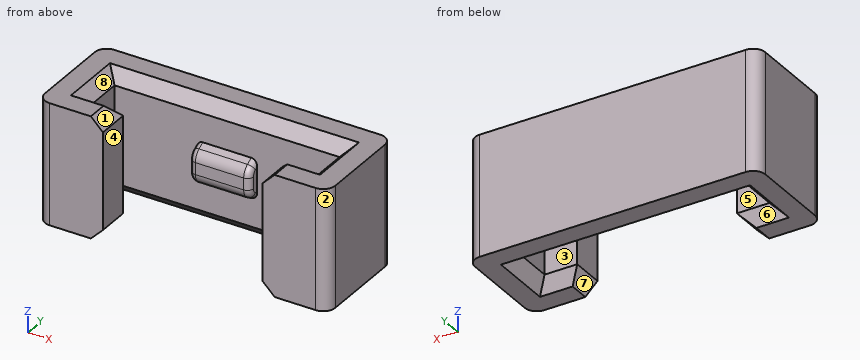
from build123d import *

# Parameters (mm, degrees)
F1_DEPTH    = 10
F2_W        = 5
F2_H        = 3.4
F3_DEPTH    = 1
F4_T4_DEPTH = 10.6915886602
F4_T9_DEPTH = 10.6915886602
F5_R        = 1
F6_R        = 0.5
F7_SIZE     = 1
F8_R        = 1


# Not quite as in the source:
# - a fillet or chamfer that OpenCascade refuses, or shapes differently, is made with other operations: its cross-section is extruded or revolved along the edge and cut away or added


with BuildPart() as f1:
    # F0 (on Top) → F1 (new body)
    with BuildSketch(Plane.XY):
        Polygon((-6.6, -5.9), (-9.3, -5.9), (-9.3, -2.7), (0, -2.7), (9.3, -2.7), (9.3, -5.9), (6.6, -5.9), (6.6, -8.6), (12, -8.6), (12, 0), (0, 0), (-12, 0), (-12, -8.6), (-6.6, -8.6), align=None)
    extrude(amount=F1_DEPTH)

    # F2 (on face) → F3 (join)
    with BuildSketch(Plane.XZ.offset(2.7)):
        with Locations((0, 5)):
            Rectangle(F2_W, F2_H)
    extrude(amount=F3_DEPTH)

    # F4: chamfer of 1.1 x 0.6350852961 on 2 edges, made by hand


with BuildPart() as f4_tool2:
    # F4_s3 → F4_t4 (new body)
    with BuildSketch(Plane.YZ.offset(5.3457943301)):
        Polygon((-2.6, 6.7), (-3.7, 6.0649147039), (-3.7, 6.7), align=None)
    extrude(amount=-F4_T4_DEPTH)

    split(bisect_by=Plane.XZ.offset(2.7), keep=Keep.TOP)


with BuildPart() as f1_1:
    add(f1.part)

    # F4_t1: cut F4_tool2
    add(f4_tool2.part, mode=Mode.SUBTRACT)


with BuildPart() as f4_tool7:
    # F4_s8 → F4_t9 (new body)
    with BuildSketch(Plane.YZ.offset(-5.3457943301)):
        Polygon((-2.6, 3.3), (-3.7, 3.9350852961), (-3.7, 3.3), align=None)
    extrude(amount=F4_T9_DEPTH)

    split(bisect_by=Plane.XZ.offset(2.7), keep=Keep.TOP)


with BuildPart() as f1_2:
    add(f1_1.part)

    # F4_t6: cut F4_tool7
    add(f4_tool7.part, mode=Mode.SUBTRACT)

    # F5
    f5_edges = [f1_2.edges().sort_by_distance(p)[0] for p in [
        (0, -3.7, 3.935085),
        (0, -3.7, 6.064915),
    ]]
    fillet(f5_edges, radius=F5_R)

    # F6
    f6_edges = [f1_2.edges().sort_by_distance(p)[0] for p in [
        (2.5, -3.566025, 4.012436),
        (2.5, -3.566025, 5.987564),
        (-2.5, -3.566025, 4.012436),
        (-2.5, -3.566025, 5.987564),
        (2.5, -2.95, 6.497927),
        (-2.5, -2.95, 6.497927),
        (2.5, -3.7, 5),
        (2.5, -2.95, 3.502073),
        (-2.5, -2.95, 3.502073),
        (-2.5, -3.7, 5),
    ]]
    fillet(f6_edges, radius=F6_R)

    # F7
    f7_edges = [f1_2.edges().sort_by_distance(p)[0] for p in [
        (-9.3, -4.3, 0),
        (0, -2.7, 0),
        (-7.95, -5.9, 0),
        (-6.6, -7.25, 0),
        (9.3, -4.3, 0),
        (7.95, -5.9, 0),
        (6.6, -7.25, 0),
        (-9.3, -4.3, 10),
        (-7.95, -5.9, 10),
        (-6.6, -7.25, 10),
        (0, -2.7, 10),
        (9.3, -4.3, 10),
        (7.95, -5.9, 10),
        (6.6, -7.25, 10),
    ]]
    chamfer(f7_edges, length=F7_SIZE)

    # F8
    f8_edges = [f1_2.edges().sort_by_distance(p)[0] for p in [
        (-12, -8.6, 5),
        (12, -8.6, 5),
        (-12, 0, 5),
        (12, 0, 5),
    ]]
    fillet(f8_edges, radius=F8_R)


solid = f1_2.part
Source: CAD feature listing. Evaluate the final solid. Frame: model axes, mm. Face numbers are marked on the shaded views. A direction names the side the tool comes from. Round coordinates to 2 decimals unless told otherwise and drop trailing zeros. Loops run counter-clockwise (first coordinate to the right, second up) from the corner with the lowest first, then second, coordinate; pieces in that order, holes last. Notation, with made-up numbers: (6.25, 75.5) -> (44.25, 75.5) arc R10 cw to (44.25, 93.5) -> close; hole circle Ø3 at (17.25, 71). An arc over 180 degrees is marked (long way). Answer as a JSON object with one key per item and string values. Group by question number.
Q1. Section query B-B (y = -4.75). Output: boundary loops of the cut face in (x, z), plus the area to 3 significant figures.
Q2. Section query C-C (z = 8.75). Output: boundary loops of the cut face in (x, y).
Q3. Access query for the marked faces 4, 5, 6, 7 and 8. Directions: +Z, -Z, +X, -X, +Y, -Y. A direction counts if a zero-diameter tool reaches every point of the face in a straight line with its end or side. Return the directions, or none.
Q4. Section query A-A (x = 8.25). Output: boundary loops of the cut face in (y, z).
Q5. Section query D-D (y = -6.25). Output: boundary loops of the cut face in (x, z), plus the area to 3 significant figures.
Q6. Ray query, line 1 (X direction, y = -6.5, z = 8.5); line 2 (X direction, y = -3.75, z = 2.75); line 3 (Y direction, x = -7.5, z = 8). Return the intervals inside material, ascending. Write a range as from..to.
Q7. Mould query, pull axis Y, two halves, no side actions, for the marked faces 1, 2 and 3. Classes: pulls with the +Y half, pulls with the -Y half, needs draft (parallel to the pull), parting line crosses it, or undercut.
Q8. Contact query for flat-ended pins moving along their axis: P1, Ø1.5, axis at x = 0.5, y = -3, coming from the -Z side; P2, Ø0.5, axis at x = 0.5, z = 5, coming from the -Y side; P3, Ø1.5, axis at x = -5, y = -2.5, coming from the +Z side; P4, Ø1, axis at x = 7.5, y = -4.5, coming from the -Z side. Output: stop coordinate, or through.
Completed:
{
 "1": {"outline": "(-12, 0) -> (-10.3, 0) -> (-9.3, 1) -> (-9.3, 9) -> (-10.3, 10) -> (-12, 10) -> close; (9.3, 1) -> (10.3, 0) -> (12, 0) -> (12, 10) -> (10.3, 10) -> (9.3, 9) -> close", "area": "52.0 mm²"},
 "2": {"outline": "(-12, -7.6) arc R1 ccw to (-11, -8.6) -> (-6.6, -8.6) -> (-6.6, -5.9) -> (-9.3, -5.9) -> (-9.3, -2.7) -> (9.3, -2.7) -> (9.3, -5.9) -> (6.6, -5.9) -> (6.6, -8.6) -> (11, -8.6) arc R1 ccw to (12, -7.6) -> (12, -1) arc R1 ccw to (11, 0) -> (-11, 0) arc R1 ccw to (-12, -1) -> close"},
 "3": {"face 4": "+Z, -Z, -Y", "face 5": "+Z, -Z", "face 6": "-Z", "face 7": "-Z, -Y", "face 8": "+Z"},
 "4": {"outline": "(-8.6, 0) -> (-6.9, 0) -> (-5.9, 1) -> (-5.9, 9) -> (-6.9, 10) -> (-8.6, 10) -> close; (-2.7, 1) -> (-1.7, 0) -> (0, 0) -> (0, 10) -> (-1.7, 10) -> (-2.7, 9) -> close"},
 "5": {"outline": "(-12, 0) -> (-10.3, 0) -> (-9.65, 0.65) -> (-6.95, 0.65) -> (-6.6, 1) -> (-6.6, 9) -> (-6.95, 9.35) -> (-9.65, 9.35) -> (-10.3, 10) -> (-12, 10) -> close; (6.6, 1) -> (6.95, 0.65) -> (9.65, 0.65) -> (10.3, 0) -> (12, 0) -> (12, 10) -> (10.3, 10) -> (9.65, 9.35) -> (6.95, 9.35) -> (6.6, 9) -> close", "area": "99.0 mm²"},
 "6": {"line 1": "-12..-6.6, 6.6..12", "line 2": "-12..-9.3, 9.3..12", "line 3": "-8.6..-5.9, -2.7..0"},
 "7": {"face 1": "needs draft", "face 2": "pulls with the -Y half", "face 3": "undercut"},
 "8": {"P1": "z = 0.55", "P2": "y = -3.7", "P3": "z = 9.95", "P4": "through"}
}
